Check sheet for the modelled part. Datum: model origin and axes. Units: mm. Round coordinates to 2 decimals unless told otherwise and drop trailing zeros. Order: outer loops, then holes, each group sorted by start corner. A loop starts at its lowest first (then second) coordinate and runs counter-clockwise, first axis right, second up.
Q1. Cross-section at A-A on x = 6. Record the cut outline in (y, z), then the cut area to 3 significant figures.
Q2. Cross-section at B-B on z = 2.7. Give the number of separate pieces and of enclosed holes in the cut face, then the cut area to 3 significant figures.
Q3. Depth check by flat-ended pin: P1, Ø1.6, axis at y = -69, z = 2, coming from the -X side; P2, Ø1.6, axis at x = -69, z = 1, coming from the +Y side (3 decimals); P3, Ø5, axis at x = 17.52, y = 81.8, coming from the +Z side; P4, Ø1, axis at y = 53, z = 1.5, coming from the +X side. Enter the tip coordinate at first touch or a pass-through.
Q4. Scan lines: probe 1 along Y at (x, z) = (7, 2.4); probe 2 along Y at (x, z) = (37.5, 2.2); probe 3 along Y at (x, z) = (67.85, 1.8) (3 decimals). Record each from-to range of solid material in increasing order.
Q5. Cross-section at D-D on x = 52. Record the cut outline in (y, z), then the cut area to 3 significant figures.
Q6. Cross-section at C-C on y = -84. Record the cut outline in (x, z), then the cut area to 3 significant figures.
from build123d import *

# Parameters (mm, degrees)
SKETCH1_W           = 139.7
SKETCH1_H           = 203.2
BOSS_EXTRUDE1_DEPTH = 3.18
SKETCH2_R           = 1.5
SKETCH2_W           = 3.18
SKETCH2_H           = 91.725
CUT_EXTRUDE1_DEPTH  = 4.18
SKETCH3_R           = 1.59
CUT_EXTRUDE2_DEPTH  = 4.18
SKETCH4_R           = 1.59
CUT_EXTRUDE3_DEPTH  = 4.18
SKETCH5_W           = 88.895716174
SKETCH5_H           = 168.56277979
BOSS_EXTRUDE2_DEPTH = 3.18
SKETCH6_W           = 20
SKETCH6_H           = 203.2
BOSS_EXTRUDE3_DEPTH = 3.18
SKETCH7_W           = 56.795
SKETCH7_H           = 3.18
CUT_EXTRUDE4_DEPTH  = 4.18
SKETCH8_W           = 133.34
SKETCH8_H           = 3.18
CUT_EXTRUDE5_DEPTH  = 4.18
SKETCH9_R           = 1.6
CUT_EXTRUDE6_DEPTH  = 4.18
SKETCH10_W          = 24.565797096
SKETCH10_H          = 10.537213664
CUT_EXTRUDE7_DEPTH  = 3.18
SKETCH11_R          = 1.59
SKETCH11_R_2        = 1.71788268
CUT_EXTRUDE8_DEPTH  = 35


with BuildPart() as part:
    # Sketch1 → Boss-Extrude1 (new body)
    with BuildSketch(Plane.XY):
        Rectangle(SKETCH1_W, SKETCH1_H)
    extrude(amount=BOSS_EXTRUDE1_DEPTH)

    # Sketch2 → Cut-Extrude1 (cut, through all)
    with BuildSketch(Plane.XY.offset(3.18)):
        with Locations((-67.85, 0)):
            Circle(SKETCH2_R)
        with Locations((67.85, 0)):
            Circle(SKETCH2_R)
        Polygon((-10, 101.6), (10, 101.6), (10, 98.42), (1.5, 98.42), (1.5, 94.42), (3.5, 94.42), (3.5, 91.42), (1.5, 91.42), (1.5, 88.42), (-1.5, 88.42), (-1.5, 91.42), (-3.5, 91.42), (-3.5, 94.42), (-1.5, 94.42), (-1.5, 98.42), (-10, 98.42), align=None)
        Polygon((-10, -101.6), (-10, -98.42), (-1.5, -98.42), (-1.5, -94.42), (-3.5, -94.42), (-3.5, -91.42), (-1.5, -91.42), (-1.5, -88.42), (1.5, -88.42), (1.5, -91.42), (3.5, -91.42), (3.5, -94.42), (1.5, -94.42), (1.5, -98.42), (10, -98.42), (10, -101.6), align=None)
        with Locations((-68.26, 55.7375)):
            Rectangle(SKETCH2_W, SKETCH2_H)
        with Locations((-68.26, -55.7375)):
            Rectangle(SKETCH2_W, SKETCH2_H)
        with Locations((68.26, -55.7375)):
            Rectangle(SKETCH2_W, SKETCH2_H)
        with Locations((68.26, 55.7375)):
            Rectangle(SKETCH2_W, SKETCH2_H)
    extrude(amount=-CUT_EXTRUDE1_DEPTH, mode=Mode.SUBTRACT)

    # Sketch3 → Cut-Extrude2 (cut, through all)
    with BuildSketch(Plane(origin=(0, 0, 0), x_dir=(-1, 0, 0), z_dir=(0, 0, -1))):
        with Locations((-35.67127699, -47.963396943)):
            Circle(SKETCH3_R)
        with Locations((-35.67127699, -30.777287406)):
            Circle(SKETCH3_R)
    extrude(amount=-CUT_EXTRUDE2_DEPTH, mode=Mode.SUBTRACT)

    # Sketch4 → Cut-Extrude3 (cut, through all)
    with BuildSketch(Plane(origin=(0, 0, 0), x_dir=(-1, 0, 0), z_dir=(0, 0, -1))):
        with Locations((-34.750723073, 80.736128989)):
            Circle(SKETCH4_R)
        with Locations((-34.750723073, 63.550019452)):
            Circle(SKETCH4_R)
        with Locations((36.249784221, 80.736128989)):
            Circle(SKETCH4_R)
        with Locations((36.249784221, 63.550019452)):
            Circle(SKETCH4_R)
        with Locations((35.983928162, -30.777287406)):
            Circle(SKETCH4_R)
        with Locations((35.983928162, -47.963396943)):
            Circle(SKETCH4_R)
        with Locations((-35.67127699, -30.777287406)):
            Circle(SKETCH4_R)
        with Locations((-35.67127699, -47.963396943)):
            Circle(SKETCH4_R)
    extrude(amount=-CUT_EXTRUDE3_DEPTH, mode=Mode.SUBTRACT)

    # Sketch5 → Boss-Extrude2 (add)
    with BuildSketch(Plane.XY.offset(3.18)):
        Rectangle(SKETCH5_W, SKETCH5_H)
    extrude(amount=-BOSS_EXTRUDE2_DEPTH)

    # Sketch6 → Boss-Extrude3 (add)
    with BuildSketch(Plane.XY.offset(3.18)):
        Rectangle(SKETCH6_W, SKETCH6_H)
    extrude(amount=-BOSS_EXTRUDE3_DEPTH)

    # Sketch7 → Cut-Extrude4 (cut, through all)
    with BuildSketch(Plane.XY.offset(3.18)):
        with Locations((-38.2725, -100.01)):
            Rectangle(SKETCH7_W, SKETCH7_H)
        with Locations((38.2725, -100.01)):
            Rectangle(SKETCH7_W, SKETCH7_H)
    extrude(amount=-CUT_EXTRUDE4_DEPTH, mode=Mode.SUBTRACT)

    # Sketch8 → Cut-Extrude5 (cut, through all)
    with BuildSketch(Plane.XY.offset(3.18)):
        with Locations((0, 100.01)):
            Rectangle(SKETCH8_W, SKETCH8_H)
    extrude(amount=-CUT_EXTRUDE5_DEPTH, mode=Mode.SUBTRACT)

    # Sketch9 → Cut-Extrude6 (cut, through all)
    with BuildSketch(Plane.XY.offset(3.18)):
        with Locations((-17.947926552, -36.205077673)):
            Circle(SKETCH9_R)
        with Locations((25.333125389, 14.525884697)):
            Circle(SKETCH9_R)
        with Locations((-22.964258499, 16.202998173)):
            Circle(SKETCH9_R)
        with Locations((9.952037888, -36.24962266)):
            Circle(SKETCH9_R)
    extrude(amount=-CUT_EXTRUDE6_DEPTH, mode=Mode.SUBTRACT)

    # Sketch10 → Cut-Extrude7 (cut)
    with BuildSketch(Plane.XY.offset(3.18)):
        with Locations((-3.359789788, -56.149532718)):
            Rectangle(SKETCH10_W, SKETCH10_H)
    extrude(amount=-CUT_EXTRUDE7_DEPTH, mode=Mode.SUBTRACT)

    # Sketch11 → Cut-Extrude8 (cut)
    with BuildSketch(Plane.XY.offset(3.18)):
        with Locations((17.523878239, 81.797398404)):
            Circle(SKETCH11_R)
        with Locations((-14.883091948, 81.797398404)):
            Circle(SKETCH11_R_2)
    extrude(amount=-CUT_EXTRUDE8_DEPTH, mode=Mode.SUBTRACT)


solid = part.part
Results found:
1. outline: (-101.6, 0) - (-61.42, 0) - (-61.42, 3.18) - (-101.6, 3.18) - close; (-50.88, 0) - (98.42, 0) - (98.42, 3.18) - (-50.88, 3.18) - close
1. area: 603 mm2
2. separate pieces: 1
2. enclosed holes: 9
2. area: 26,100 mm2
3. P1: stops at x = -66.67
3. P2: stops at y = 9.875
3. P3: stops at z = 3.18
3. P4: stops at x = 66.67
4. probe 1: y = -101.6 to -61.42, -50.88 to 98.42
4. probe 2: y = -98.42 to 98.42
4. probe 3: y = -9.875 to -1.5, 1.5 to 9.875
5. outline: (-98.42, 0) - (98.42, 0) - (98.42, 3.18) - (-98.42, 3.18) - close
5. area: 626 mm2
6. outline: (-66.67, 0) - (66.67, 0) - (66.67, 3.18) - (-66.67, 3.18) - close
6. area: 424 mm2
